Geometry: final body of the model. Coordinates: model frame, mm. A direction names the side the tool comes from. Round coordinates to 2 decimals unless told otherwise and drop trailing zeros. Loops run counter-clockwise (first coordinate to the right, second up) from the corner with the lowest first, then second, coordinate; pieces in that order, holes last. Notation, with made-up numbers: (1.5, -0.75) -> (56.5, -0.75) arc R26 ccw to (56.5, 18.25) -> close; hole circle Ø8 at (46.25, 24.25). An arc over 180 degrees is marked (long way). Answer in a Markdown table with one row per item.
```python
from build123d import *

# Parameters (mm, degrees)
ESQUISSE1_W             = 23.2
ESQUISSE1_H             = 12.5
BOSS_EXTRU_1_DEPTH      = 23
ESQUISSE2_W             = 4.7
ESQUISSE2_H             = 2.4
BOSS_EXTRU_2_DEPTH      = 12.5
CONG_1_R                = 0.75
ESQUISSE3_R             = 2.5
ENL_V_MAT_EXTRU_1_DEPTH = 11.8
CONG_2_R                = 0.2
CONG_3_R                = 0.5
ESQUISSE5_R             = 6
BOSS_EXTRU_3_DEPTH      = 4.3
ESQUISSE6_R             = 1.461217274
BOSS_EXTRU_4_DEPTH      = 2.5


with BuildPart() as part:
    # Esquisse1 → Boss.-Extru.1 (new body)
    with BuildSketch(Plane(origin=(0, 0, 0), x_dir=(1, 0, 0), z_dir=(0, 1, 0))):
        Rectangle(ESQUISSE1_W, ESQUISSE1_H)
    extrude(amount=BOSS_EXTRU_1_DEPTH)

    # Esquisse2 → Boss.-Extru.2 (add)
    with BuildSketch(Plane.XY.offset(6.25)):
        with Locations((13.95, 17.6)):
            Rectangle(ESQUISSE2_W, ESQUISSE2_H)
        with Locations((-13.95, 17.6)):
            Rectangle(ESQUISSE2_W, ESQUISSE2_H)
    extrude(amount=-BOSS_EXTRU_2_DEPTH)

    # Congé1
    cong_1_edges = [part.edges().sort_by_distance(p)[0] for p in [
        (16.3, 17.6, -6.25),
        (16.3, 17.6, 6.25),
        (-16.3, 17.6, -6.25),
        (-16.3, 17.6, 6.25),
    ]]
    fillet(cong_1_edges, radius=CONG_1_R)

    # Esquisse3 → Enlèv. mat.-Extru.1 (cut)
    with BuildSketch(Plane(origin=(0, 23, 0), x_dir=(1, 0, 0), z_dir=(0, 1, 0))):
        with Locations((-14.5, 0)):
            Circle(ESQUISSE3_R)
        with Locations((14.5, 0)):
            Circle(ESQUISSE3_R)
    extrude(amount=-ENL_V_MAT_EXTRU_1_DEPTH, mode=Mode.SUBTRACT)

    # Congé2
    cong_2_edges = [part.edges().sort_by_distance(p)[0] for p in [
        (-16.3, 17.6, -1.734935157),
        (-16.3, 17.6, 1.734935157),
        (16.3, 17.6, -1.734935157),
        (16.3, 17.6, 1.734935157),
    ]]
    fillet(cong_2_edges, radius=CONG_2_R)

    # Congé3
    cong_3_edges = [part.edges().sort_by_distance(p)[0] for p in [
        (11.6, 8.2, -6.25),
        (11.6, 8.2, 6.25),
        (-11.6, 8.2, 6.25),
        (-11.6, 8.2, -6.25),
        (11.6, 20.9, 6.25),
        (-11.6, 20.9, 6.25),
        (-11.6, 20.9, -6.25),
        (11.6, 20.9, -6.25),
    ]]
    fillet(cong_3_edges, radius=CONG_3_R)

    # Esquisse5 → Boss.-Extru.3 (add)
    with BuildSketch(Plane(origin=(0, 23, 0), x_dir=(1, 0, 0), z_dir=(0, 1, 0))):
        with Locations((5.6, 0)):
            Circle(ESQUISSE5_R)
    extrude(amount=BOSS_EXTRU_3_DEPTH)

    # Esquisse6 → Boss.-Extru.4 (add)
    with BuildSketch(Plane(origin=(0, 27.3, 0), x_dir=(1, 0, 0), z_dir=(0, 1, 0))):
        with Locations(Location((5.6, 0, 0), (0, 0, 270))):
            Circle(ESQUISSE6_R)
    extrude(amount=BOSS_EXTRU_4_DEPTH)


solid = part.part
```
Item 1: Set-up query: faces 1 (the flat face through (7, 27.3, 1)), 2 (the flat face through (0, 0, 0)), 3 (the flat face through (-11.6, 8, 0)), 4 (the flat face through (11.6, 21, 0)), 5 (the flat face through (-11.6, 21, 0)). Return all of +Z, -Z, +X, -X, +Y, -Y with unobstructed straight access to the full face (end or side cutting, diameter ignored); none if empty.
Ans:
| item | result |
|---|---|
| face 1 | +Y |
| face 2 | +Z, -Z, +X, -X, -Y |
| face 3 | +Z, -Z, -X, -Y |
| face 4 | +Z, -Z, +X, +Y |
| face 5 | +Z, -Z, -X, +Y |
Item 2: Section query C-C, the plane x = -14.5. Output: boundary loops of the cut face in (y, z), and give its area (3 significant figures).
Ans:
| item | result |
|---|---|
| outline | (16.4, -6.25) -> (18.8, -6.25) -> (18.8, -2.5) -> (16.4, -2.5) -> close; (16.4, 2.5) -> (18.8, 2.5) -> (18.8, 6.25) -> (16.4, 6.25) -> close |
| area | 18.0 mm2 |
Item 3: Ray query, L1, parallel to Z at x = 14.5, y = 17.8; L2, parallel to X at y = 18.5, z = 2.25; L3, parallel to Y at x = -10.5, z = -2.5. Return the intervals inside material, ascending.
Ans:
| item | result |
|---|---|
| L1 | -6.25 to -2.5, 2.5 to 6.25 |
| L2 | -16.3 to -15.59, -13.41 to 13.41, 15.59 to 16.3 |
| L3 | 0 to 23 |
Item 4: Section query B-B, the plane y = 8.25. Output: boundary loops of the cut face in (x, z).
Ans:
| item | result |
|---|---|
| outline | (-11.6, -5.75) arc R0.5 ccw to (-11.1, -6.25) -> (11.1, -6.25) arc R0.5 ccw to (11.6, -5.75) -> (11.6, 5.75) arc R0.5 ccw to (11.1, 6.25) -> (-11.1, 6.25) arc R0.5 ccw to (-11.6, 5.75) -> close |
Item 5: Mould query, pull axis Z, two halves, no side actions, for faces 6 (the cylindrical face through (4.174, 28.532, -0.317)), 7 (the flat face through (11.6, 8, 0)), 8 (the cylindrical face through (12, 18, 0)). Classes: released by +Z, released by -Z, zero draft, split by the parting line, or undercut.
Ans:
| item | result |
|---|---|
| face 6 | split by the parting line |
| face 7 | zero draft |
| face 8 | undercut |
Item 6: Section query D-D, the plane z = -3. Output: boundary loops of the cut face in (x, y), and give its area (3 significant figures).
Ans:
| item | result |
|---|---|
| outline | (-16.3, 16.4) -> (-11.6, 16.4) -> (-11.6, 0) -> (11.6, 0) -> (11.6, 16.4) -> (16.3, 16.4) -> (16.3, 18.8) -> (11.6, 18.8) -> (11.6, 23) -> (10.8, 23) -> (10.8, 27.3) -> (0.4, 27.3) -> (0.4, 23) -> (-11.6, 23) -> (-11.6, 18.8) -> (-16.3, 18.8) -> close |
| area | 601 mm2 |
Item 7: Section query A-A, the plane x = 12.5. Output: boundary loops of the cut face in (y, z).
Ans:
| item | result |
|---|---|
| outline | (16.4, -6.25) -> (18.8, -6.25) -> (18.8, -1.5) -> (16.4, -1.5) -> close; (16.4, 1.5) -> (18.8, 1.5) -> (18.8, 6.25) -> (16.4, 6.25) -> close |
Item 8: First-contact query: P1, Ø3.5, axis at y = 10, z = 0.5, coming from the -X side; P2, Ø2.5, axis at x = -13, z = 1.5, coming from the +Y side; P3, Ø2, axis at y = 21, z = -0.5, coming from the +X side. Flat tips, straight axial feed; report the tip coordinate or a pass-through.
Ans:
| item | result |
|---|---|
| P1 | x = -11.6 |
| P2 | y = 18.8 |
| P3 | x = 11.6 |
